```python
from build123d import *

# Parameters (mm, degrees)
CROQUIS1_R              = 11
SALIENTE_EXTRUIR1_DEPTH = 21.4
CROQUIS2_R              = 2
SALIENTE_EXTRUIR2_DEPTH = 15.3
CROQUIS3_R              = 9
SALIENTE_EXTRUIR3_DEPTH = 18


with BuildPart() as part:
    # Croquis1 → Saliente-Extruir1 (new body)
    with BuildSketch(Plane(origin=(0, 0, 0), x_dir=(1, 0, 0), z_dir=(0, 1, 0))):
        Circle(CROQUIS1_R)
    extrude(amount=SALIENTE_EXTRUIR1_DEPTH)

    # Croquis2 → Saliente-Extruir2 (add)
    with BuildSketch(Plane(origin=(0, 21.4, 0), x_dir=(1, 0, 0), z_dir=(0, 1, 0))):
        Circle(CROQUIS2_R)
    extrude(amount=SALIENTE_EXTRUIR2_DEPTH)

    # Croquis3 → Saliente-Extruir3 (add)
    with BuildSketch(Plane.XZ):
        Circle(CROQUIS3_R)
    extrude(amount=SALIENTE_EXTRUIR3_DEPTH)


solid = part.part
```
Part model, mm, in its own coordinate system. A direction names the side the tool comes from. Round coordinates to 2 decimals unless told otherwise and drop trailing zeros. Write each loop counter-clockwise with the first axis right and the second up, starting at its lowest first coordinate (ties: lowest second). Pieces come first, ordered by that corner, then holes.
Item 1: Which spindle directions (+Z, -Z, +X, -X, +Y, -Y) get a long thin tool onto all of the face, cutting with end or side? Do faces 1 (the flat face through (0, -18, 0)), 2 (the cylindrical face through (0, 29, 2)), 3 (the cylindrical face through (-1.172, -8.874, 8.923)). Say none if no direction does.
Results:
face 1: +Z, -Z, +X, -X, -Y
face 2: +Y
face 3: -Y
Item 2: Cut at B-B, the plane z = 8. Give the cut face in (x, y), plus the area to 3 significant figures.
Results:
outline: (-7.55, 0) - (-4.12, 0) - (-4.12, -18) - (4.12, -18) - (4.12, 0) - (7.55, 0) - (7.55, 21.4) - (-7.55, 21.4) - close
area: 472 mm2
Item 3: Probe L1, parallel to Y at x = 9.5, z = -2.25; L2, parallel to Y at x = 2, z = -3.25; L3, parallel to X at y = 20.5, z = 0.25. List the from-to ranges inside material, lowest first.
Results:
L1: y = 0 to 21.4
L2: y = -18 to 21.4
L3: x = -11 to 11
Item 4: Drop flat-ended pins along their axis: pin 1 Ø1 at (x, z) = (1, -4) entering from +Y; pin 2 Ø3 at (y, z) = (1, -4.5) entering from +X; pin 3 Ø10 at (y, z) = (-11, -5) entering from -X. Give the stop position or say it passes through.
Results:
pin 1: stops at y = 21.4
pin 2: stops at x = 10.58
pin 3: stops at x = -9
Item 5: Cut at C-C, the plane y = -12.5. Give the cut face in (x, z).
Results:
outline: circle Ø18 at (0, 0)
Item 6: Cut at D-D, the plane z = 0. Give the cut face in (x, y), plus the area to 3 significant figures.
Results:
outline: (-11, 0) - (-9, 0) - (-9, -18) - (9, -18) - (9, 0) - (11, 0) - (11, 21.4) - (2, 21.4) - (2, 36.7) - (-2, 36.7) - (-2, 21.4) - (-11, 21.4) - close
area: 856 mm2
Item 7: Cut at A-A, the plane x = 0. Give the cut face in (y, z).
Results:
outline: (-18, -9) - (0, -9) - (0, -11) - (21.4, -11) - (21.4, -2) - (36.7, -2) - (36.7, 2) - (21.4, 2) - (21.4, 11) - (0, 11) - (0, 9) - (-18, 9) - close
